Verification items for this drawing (mm, ordinates from the low corner). Round coordinates to 2 decimals unless told otherwise and drop trailing zeros. Loops run counter-clockwise (first coordinate to the right, second up) from the corner with the lowest first, then second, coordinate; pieces in that order, holes last. Notation, with made-up numbers: (50, -22) -> (59, -22) arc R21 cw to (59, 7) -> close; hole circle Ø7 at (-27.5, -36.5). An arc over 180 degrees is marked (long way). Use a Markdown table: item, result. Add a question column.
Q1. Sectioned sample at A-A, the plane z = 4.25. Enter the section's corners in (x, y).
Q2. Sectioned sample at B-B, the plane y = 20.5. Enter the section's corners in (x, z) (1 decimal).
Q3. Gauge pin test, flat ends, axial feed: P1, Ø1, axis at x = 43.5, z = 14.5, coming from the -Y side; P2, Ø8, axis at y = 72.5, z = 17, coming from the -X side; P3, Ø8, axis at y = 85, z = 4, coming from the +X side; P4, Ø5, axis at y = 41, z = 20.5, coming from the +X side. Record the tip position at first contact, or that the pin passes through.
Q4. Sectioned sample at C-C, the plane x = 39.5. Enter the section's corners in (y, z) (1 decimal), then the cut area to 3 significant figures.
Q5. Material ranges on L1, parallel to X at y = 72.5, z = 2.25; L2, parallel to X at y = 85.5, z = 12, recorded low to high.
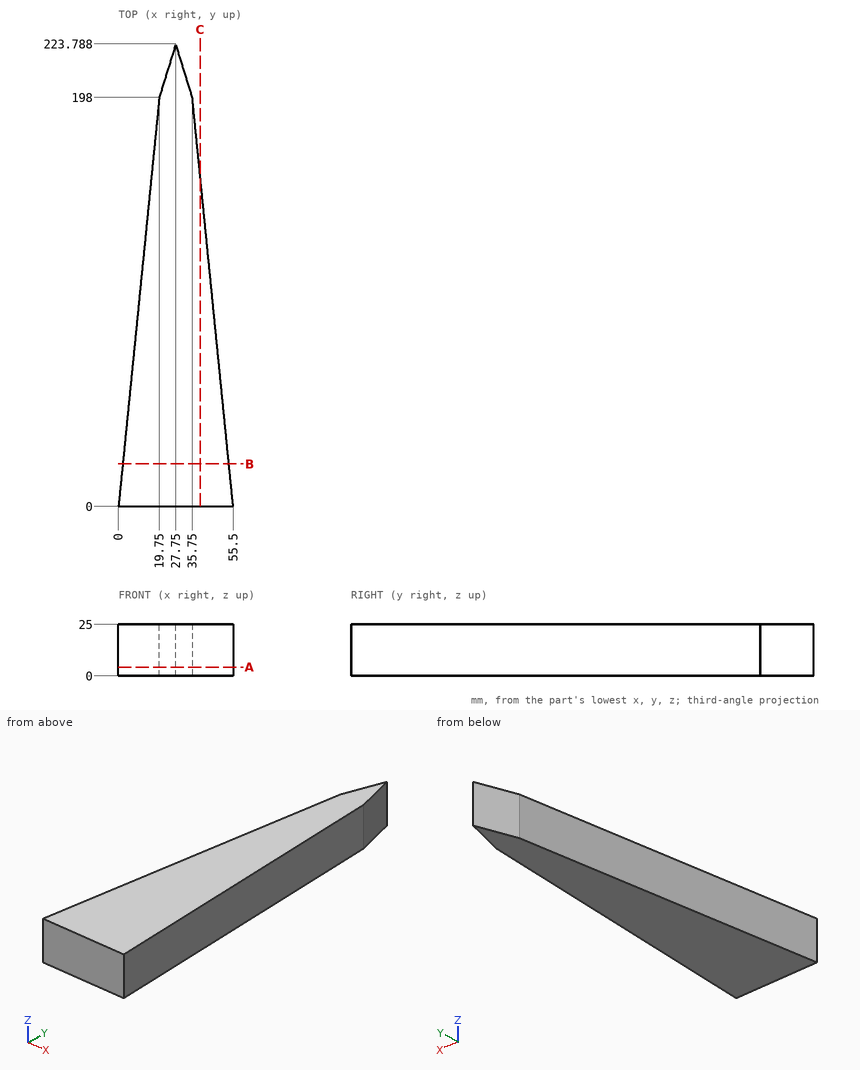
Values:
| question | item | result |
|---|---|---|
| 1 | outline | (0, 0) -> (55.5, 0) -> (35.75, 198) -> (27.75, 223.79) -> (19.75, 198) -> close |
| 2 | outline | (2, 0) -> (53.5, 0) -> (53.5, 25) -> (2, 25) -> close |
| 3 | P1 | y = 0 |
| 3 | P2 | x = 6.83 |
| 3 | P3 | x = 47.42 |
| 3 | P4 | x = 51.66 |
| 4 | outline | (0, 0) -> (160.4, 0) -> (160.4, 25) -> (0, 25) -> close |
| 4 | area | 4,010 mm^2 |
| 5 | L1 | 7.23 to 48.27 |
| 5 | L2 | 8.53 to 46.97 |
